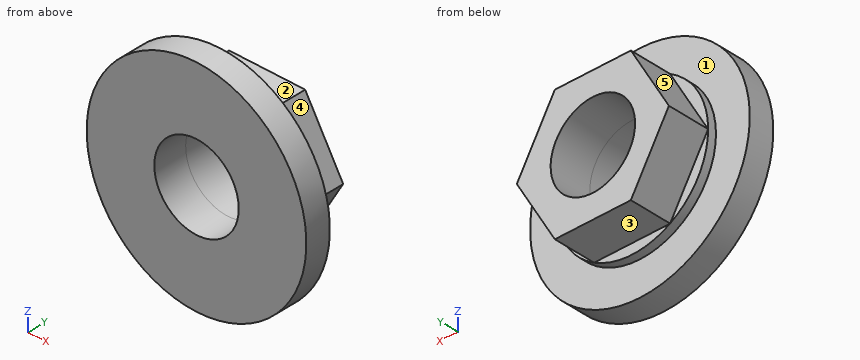
```python
from build123d import *

# Parameters (mm, degrees)
SKETCH1_R           = 6.5
BOSS_EXTRUDE1_DEPTH = 1.5
SKETCH2_R           = 4.5
BOSS_EXTRUDE2_DEPTH = 0.5
SKETCH3_R           = 2.5
BOSS_EXTRUDE3_DEPTH = 2.5
SKETCH4_R           = 2.5
CUT_EXTRUDE1_DEPTH  = 3.5


with BuildPart() as part:
    # Sketch1 → Boss-Extrude1 (new body)
    with BuildSketch(Plane(origin=(0, 0, 0), x_dir=(1, 0, 0), z_dir=(0, 1, 0))):
        with Locations(Location((0, 0, 0), (0, 0, 270))):  # turned: the seam where the file's is
            Circle(SKETCH1_R)
    extrude(amount=BOSS_EXTRUDE1_DEPTH)

    # Sketch2 → Boss-Extrude2 (add)
    with BuildSketch(Plane(origin=(0, 1.5, 0), x_dir=(1, 0, 0), z_dir=(0, 1, 0))):
        with Locations(Location((0, 0, 0), (0, 0, 270))):  # turned: the seam where the file's is
            Circle(SKETCH2_R)
    extrude(amount=BOSS_EXTRUDE2_DEPTH)

    # Sketch3 → Boss-Extrude3 (add)
    with BuildSketch(Plane(origin=(0, 2, 0), x_dir=(1, 0, 0), z_dir=(0, 1, 0))):
        Polygon((-4.5, 0), (-2.25, -3.897114317), (2.25, -3.897114317), (4.5, 0), (2.25, 3.897114317), (-2.25, 3.897114317), align=None)
        with Locations(Location((0, 0, 0), (0, 0, 270))):  # turned: the seam where the file's is
            Circle(SKETCH3_R, mode=Mode.SUBTRACT)
    extrude(amount=BOSS_EXTRUDE3_DEPTH)

    # Sketch4 → Cut-Extrude1 (cut)
    with BuildSketch(Plane(origin=(0, 2, 0), x_dir=(1, 0, 0), z_dir=(0, 1, 0))):
        with Locations(Location((0, 0, 0), (0, 0, 270))):  # turned: the seam where the file's is
            Circle(SKETCH4_R)
    extrude(amount=-CUT_EXTRUDE1_DEPTH, mode=Mode.SUBTRACT)


solid = part.part
```
Part model, mm, in its own coordinate system. Face numbers are marked on the shaded views. A direction names the side the tool comes from. Round coordinates to 2 decimals unless told otherwise and drop trailing zeros. Order: outer loops, then holes, each group sorted by start corner. A loop starts at its lowest first (then second) coordinate and runs counter-clockwise, first axis right, second up. Notation, with made-up numbers: M -20,-11.5 L 39,-11.5 A23 ccw 39,-1.5 Z; hole C 43,40.25 d3. An arc over 180 degrees is marked long. Answer in a Markdown table with one row per item. Add a question column.
Q1. Cut at A-A on x = 0. Give the cut face in (y, z).
Q2. Cut at B-B on y = 4.25. Give the cut face in (x, z).
Q3. 3-axis set-ups, long thin cutter, end or side, ignore diameter. For the marked faces 1, 2, 3, 4 and 5: which of +Z, -Z, +X, -X, +Y, -Y reach the whole face in a straight line?
Q4. Cut at C-C on z = 1. Give the cut face in (x, y), and give its area (3 significant figures).
Q5. Cut at D-D on z = 4.75. Give the cut face in (x, y).
Q6. Pin check, flat tips, straight feed: pin 1 (1.8 mm diameter, centred on x = 4, z = -1.5, fed in from +Y); pin 2 (3 mm diameter, centred on x = 5, z = 2.5, fed in from +Y); pin 3 (2 mm diameter, centred on x = -0.5, y = 3.5, fed in from -Z); pin 4 (3 mm diameter, centred on x = 0, z = 0, fed in from +Y). Stop position of each tip, or through.
Q7. Wall check: L1, parallel to X at y = 1.3, z = 0; L2, parallel to Y at x = -2.75, z = 5.5; L3, parallel to X at y = 1, z = -0.75. Give the ranges that are in metal, low to high. Write a range as from..to.
Established:
| question | item | result |
|---|---|---|
| 1 | outline | M 0,-6.5 L 1.5,-6.5 L 1.5,-4.5 L 2,-4.5 L 2,-3.9 L 4.5,-3.9 L 4.5,-2.5 L 0,-2.5 Z; M 0,2.5 L 4.5,2.5 L 4.5,3.9 L 2,3.9 L 2,4.5 L 1.5,4.5 L 1.5,6.5 L 0,6.5 Z |
| 2 | outline | M -4.5,0 L -2.25,-3.9 L 2.25,-3.9 L 4.5,0 L 2.25,3.9 L -2.25,3.9 Z; hole C 0,0 d5 |
| 3 | face 1 | +Y |
| 3 | face 2 | +Z, +X, -X, +Y |
| 3 | face 3 | -Z, +X, -X, +Y |
| 3 | face 4 | +Z, +X, +Y |
| 3 | face 5 | +Z, -X, +Y |
| 4 | outline | M -6.42,0 L -2.29,0 L -2.29,4.5 L -3.92,4.5 L -3.92,2 L -4.39,2 L -4.39,1.5 L -6.42,1.5 Z; M 2.29,0 L 6.42,0 L 6.42,1.5 L 4.39,1.5 L 4.39,2 L 3.92,2 L 3.92,4.5 L 2.29,4.5 Z |
| 4 | area | 22.6 mm2 |
| 5 | outline | M -4.44,0 L 4.44,0 L 4.44,1.5 L -4.44,1.5 Z |
| 6 | pin 1 | stops at y = 4.5 |
| 6 | pin 2 | stops at y = 2 |
| 6 | pin 3 | stops at z = -3.9 |
| 6 | pin 4 | passes through |
| 7 | L1 | x = -6.5..-2.5, 2.5..6.5 |
| 7 | L2 | y = 0..1.5 |
| 7 | L3 | x = -6.46..-2.38, 2.38..6.46 |
